from build123d import *

# Parameters (mm, degrees)
SKETCH1_R           = 9
SKETCH1_R_2         = 6.9
BOSS_EXTRUDE1_DEPTH = 10
SKETCH2_W           = 4
SKETCH2_H           = 7.765292285
CUT_EXTRUDE1_DEPTH  = 14
SKETCH3_W           = 2.178666284
SKETCH3_H           = 14.18086127
SKETCH3_W_2         = 2.164116959
SKETCH3_H_2         = 14.122068743
BOSS_EXTRUDE2_DEPTH = 10
SKETCH4_W           = 2.178666284
SKETCH4_H           = 7.791069301
SKETCH4_W_2         = 2.164116959
BOSS_EXTRUDE3_DEPTH = 18
SKETCH5_W           = 23.023428876
SKETCH5_H           = 2.946570651
CUT_EXTRUDE2_DEPTH  = 18
SKETCH6_R           = 37.134957589
CUT_EXTRUDE3_DEPTH  = 0.5
FILLET1_R           = 0.5
FILLET2_R           = 0.5
FILLET3_R           = 0.5


with BuildPart() as part:
    # Sketch1 → Boss-Extrude1 (new body)
    with BuildSketch(Plane(origin=(0, 0, 0), x_dir=(1, 0, 0), z_dir=(0, 1, 0))):
        with Locations(Location((0, 0, 0), (0, 0, 270))):
            Circle(SKETCH1_R)
        with Locations(Location((0, 0, 0), (0, 0, 270))):
            Circle(SKETCH1_R_2, mode=Mode.SUBTRACT)
    extrude(amount=BOSS_EXTRUDE1_DEPTH)

    # Sketch2 → Cut-Extrude1 (cut)
    with BuildSketch(Plane(origin=(0, 10, 0), x_dir=(1, 0, 0), z_dir=(0, 1, 0))):
        with Locations((0.097051884, -9.080757725)):
            Rectangle(SKETCH2_W, SKETCH2_H)
    extrude(amount=-CUT_EXTRUDE1_DEPTH, mode=Mode.SUBTRACT)

    # Sketch3 → Boss-Extrude2 (add)
    with BuildSketch(Plane(origin=(0, 10, 0), x_dir=(1, 0, 0), z_dir=(0, 1, 0))):
        with Locations((3.186385026, -13.664042534)):
            Rectangle(SKETCH3_W, SKETCH3_H)
        with Locations((-2.985006596, -13.693438798)):
            Rectangle(SKETCH3_W_2, SKETCH3_H_2)
    extrude(amount=-BOSS_EXTRUDE2_DEPTH)

    # Sketch4 → Boss-Extrude3 (add)
    with BuildSketch(Plane(origin=(0, -13.970289025, 0), x_dir=(1, 0, 0), z_dir=(0, 1, 0))):
        with Locations((3.186385026, -16.858938519)):
            Rectangle(SKETCH4_W, SKETCH4_H)
        with Locations((-2.985006596, -16.858938519)):
            Rectangle(SKETCH4_W_2, SKETCH4_H)
    extrude(amount=BOSS_EXTRUDE3_DEPTH)

    # Sketch5 → Cut-Extrude2 (cut)
    with BuildSketch(Plane(origin=(0, 0, 0), x_dir=(-1, 0, 0), z_dir=(0, -1, 0))):
        with Locations((7.23599627, -14.436689194)):
            Rectangle(SKETCH5_W, SKETCH5_H)
    extrude(amount=CUT_EXTRUDE2_DEPTH, mode=Mode.SUBTRACT)

    # Sketch6 → Cut-Extrude3 (cut)
    with BuildSketch(Plane.XY.offset(20.754473169)):
        with Locations((-4.067065075, 10)):
            Circle(SKETCH6_R)
    extrude(amount=-CUT_EXTRUDE3_DEPTH, mode=Mode.SUBTRACT)

    # Fillet1
    fillet1_edges = [part.edges().sort_by_distance(p)[0] for p in [
        (-2.985006595, -13.970289025, 15.909974519),
        (3.186385026, -13.970289025, 15.909974519),
        (3.186385026, 10, 20.254473169),
        (-2.985006595, 10, 20.254473169),
        (3.186385026, -13.970289025, 20.254473169),
        (-2.985006595, -13.970289025, 20.254473169),
    ]]
    fillet(fillet1_edges, radius=FILLET1_R)

    # Fillet2
    fillet2_edges = [part.edges().sort_by_distance(p)[0] for p in [
        (-0.117739094, 0, -8.999229828),
    ]]
    fillet(fillet2_edges, radius=FILLET2_R)

    # Fillet3
    fillet3_edges = [part.edges().sort_by_distance(p)[0] for p in [
        (-0.101406156, 10, -6.8992548),
    ]]
    fillet(fillet3_edges, radius=FILLET3_R)


solid = part.part
Can you work these out from the model? Positions are in its coordinate system, mm. A direction names the side the tool comes from. Coordinates: 2 decimals unless noted, no trailing zeros. Write each loop counter-clockwise with the first axis right and the second up, starting at its lowest first coordinate (ties: lowest second). Pieces come first, ordered by that corner, then holes. Notation, with made-up numbers: (60, -26.75) - (92, -26.75) arc R25 cw to (92, -3.75) - close; hole circle Ø10 at (79.5, 34). An arc over 180 degrees is marked (long way). Return JSON: item names as keys, results as strings. Group by question number.
Item 1: If we section it at D-D (z = 0): Write out the boundary of the cut face in (x, y), then the cut area to 3 significant figures.
Item 2: We'd pull the mould along X, two halves only. Please class faces 3 (the face through (2.097, 1, 15)), 4 (the face through (3, -2, 20.254)), 5 (the face through (-1.903, 1, 15)), 6 (the face through (4.276, 1, 15)): pulls with the +X half, pulls with the -X half, needs draft (parallel to the pull), parting line crosses it, or undercut.
Item 3: If we section it at C-C (x = 0): Write out the boundary of the cut face in (y, z), then the cut area to 3 significant figures.
Item 4: I'm going to push flat-ended pins straight in: pin 1 Ø10 at (y, z) = (-4, 15.5) entering from -X; pin 2 Ø14 at (y, z) = (2, 14.5) entering from +X; pin 3 Ø1 at (x, z) = (-4.5, 13) entering from -Y. Where does each tip first touch, or does it pass through?
Item 5: If we section it at B-B (y = -7.5): Write out the boundary of the cut face in (x, z).
Item 6: Which directions (+Z, -Z, +X, -X, +Y, -Y) give clear straight access to the entire face, cutting with the end or side of a thin tool? Please do faces 1 (the face through (-3, -7, 15.91)), 2 (the face through (3, -13.97, 18)).
Item 7: Please list where these lines run through material, in increasing order: probe 1 along X at (y, z) = (6.25, 0); probe 2 along X at (y, z) = (-12.75, 16.5); probe 3 along Y at (x, z) = (2.25, 13).
Item 8: If we section it at A-A (z = 17.75): Write out the boundary of the cut face in (x, y), then the cut area to 3 significant figures.
Return value:
{
 "1": {"outline": "(-9, 0.5) arc R0.5 ccw to (-8.5, 0) - (-6.9, 0) - (-6.9, 9.5) arc R0.5 ccw to (-7.4, 10) - (-9, 10) - close; (6.9, 0) - (8.5, 0) arc R0.5 ccw to (9, 0.5) - (9, 10) - (7.4, 10) arc R0.5 ccw to (6.9, 9.5) - close", "area": "41.8 mm^2"},
 "2": {"face 3": "undercut", "face 4": "needs draft", "face 5": "undercut", "face 6": "pulls with the +X half"},
 "3": {"outline": "(0, -8.5) arc R0.5 ccw to (0.5, -9) - (10, -9) - (10, -7.4) arc R0.5 ccw to (9.5, -6.9) - (0, -6.9) - close", "area": "20.9 mm^2"},
 "4": {"pin 1": "stops at x = -4.07", "pin 2": "stops at x = 4.97", "pin 3": "stops at y = 0"},
 "5": {"outline": "(-4.07, 15.91) - (-1.9, 15.91) - (-1.9, 20.25) - (-4.07, 20.25) - close; (2.1, 15.91) - (4.28, 15.91) - (4.28, 20.25) - (2.1, 20.25) - close"},
 "6": {"face 1": "-Z, +X, -X, -Y", "face 2": "+Z, -Z, +X, -X, -Y"},
 "7": {"probe 1": "x = -9 to -6.9, 6.9 to 9", "probe 2": "x = -4.07 to -1.9, 2.1 to 4.28", "probe 3": "y = 0 to 10"},
 "8": {"outline": "(-4.07, -13.97) - (-1.9, -13.97) - (-1.9, 10) - (-4.07, 10) - close; (2.1, -13.97) - (4.28, -13.97) - (4.28, 10) - (2.1, 10) - close", "area": "104 mm^2"}
}
